Could you check a few things on this model? Use its own coordinates, in mm. Face numbers are marked on the shaded views. A direction names the side the tool comes from. Coordinates: 2 decimals unless noted, no trailing zeros. Loops run counter-clockwise (first coordinate to the right, second up) from the corner with the lowest first, then second, coordinate; pieces in that order, holes last. Notation, with made-up numbers: M 6.5,37 L 19.5,37 A20 cw 19.5,58 Z; hole C 73,-3.5 d7. An arc over 180 degrees is marked long. Write each question's results on one line, items separated by ' | '.
```python
from build123d import *

# Parameters (mm, degrees)
BASE_FLANGE1_DEPTH = 550
SKETCH10_R         = 3
CUT_EXTRUDE2_DEPTH = 10


# Sheet-metal steps are written as plain solids
with BuildPart() as part:
    # Sketch1 → Base-Flange1 (new body)
    with BuildSketch(Plane.XY):
        with BuildLine():
            Line((0, 0), (29.2634, 0))
            ThreePointArc((29.2634, 0), (29.784254855, 0.215745145), (30, 0.7366))
            Line((30, 0.7366), (30, 200))
            Line((30, 200), (32, 200))
            Line((32, 200), (32, 0.7366))
            ThreePointArc((32, 0.7366), (31.198468417, -1.198468417), (29.2634, -2))
            Line((29.2634, -2), (0, -2))
            Line((0, -2), (0, 0))
        make_face()
    extrude(amount=BASE_FLANGE1_DEPTH)

    # Sketch10 → Cut-Extrude2 (cut)
    with BuildSketch(Plane(origin=(32, 0, 0), x_dir=(0, 0, -1), z_dir=(1, 0, 0))):
        with Locations((-50, 58)):
            Circle(SKETCH10_R)
        with Locations((-110, 58)):
            Circle(SKETCH10_R)
        with Locations((-170, 58)):
            Circle(SKETCH10_R)
        with Locations((-230, 58)):
            Circle(SKETCH10_R)
        with Locations((-290, 58)):
            Circle(SKETCH10_R)
        with Locations((-350, 58)):
            Circle(SKETCH10_R)
        with Locations((-410, 58)):
            Circle(SKETCH10_R)
    extrude(amount=-CUT_EXTRUDE2_DEPTH, mode=Mode.SUBTRACT)


solid = part.part
```
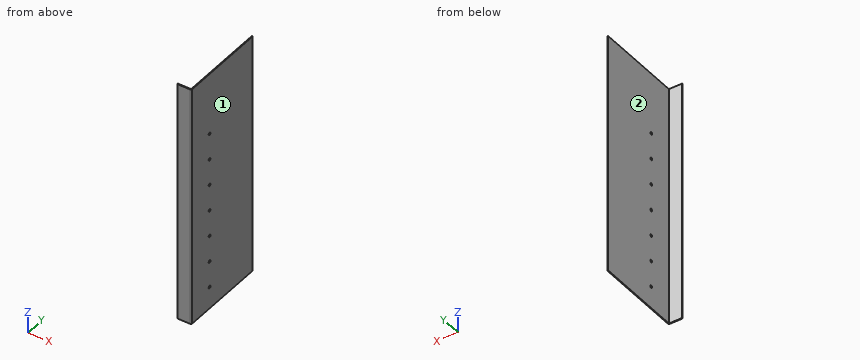
(1) Which directions (+Z, -Z, +X, -X, +Y, -Y) give clear straight access to the entire face, cutting with the end or side of a thin tool? Please do the marked faces 1 and 2.
Reported:
face 1: +Z, -Z, +X, +Y, -Y | face 2: +Z, -Z, -X, +Y
(2) Imagine slicing it at B-B, the plane y = 157. List the corners of the cut face in (x, z) for me.
Reported:
outline: M 30,0 L 32,0 L 32,550 L 30,550 Z
(3) Please list where these lines run through material, in increasing order: probe 1 along Y at (x, z) = (23.5, 193); probe 2 along X at (y, z) = (121, 349); probe 3 along Y at (x, z) = (31, 290). Write a range as from..to.
Reported:
probe 1: y = -2..0 | probe 2: x = 30..32 | probe 3: y = -1.38..55, 61..200
(4) Imagine slicing it at A-A, the plane z = 483. List the corners of the cut face in (x, y) for me, and give its area (3 significant figures).
Reported:
outline: M 0,-2 L 29.26,-2 A2.74 ccw 32,0.74 L 32,200 L 30,200 L 30,0.74 A0.74 cw 29.26,0 L 0,0 Z | area: 463 mm2
(5) Will these pins go through, and if not, where does the flat tip stop? P1, Ø2, axis at x = 14, z = 248, coming from the +Y side; P2, Ø3.5, axis at y = 58, z = 410, coming from the +X side; P3, Ø6, axis at y = 148, z = 343.5, coming from the -X side.
Reported:
P1: stops at y = 0 | P2: passes through | P3: stops at x = 30
(6) Imagine slicing it at C-C, the plane x = 8. List the corners of the cut face in (y, z) for me.
Reported:
outline: M -2,0 L 0,0 L 0,550 L -2,550 Z
